from build123d import *

# Parameters (mm, degrees)
BOSS_EXTRUDE1_DEPTH     = 5
SKETCH3_R               = 2.39
BOSS_EXTRUDE2_DEPTH     = 23.4
MIRROR3_COPY_1_SKETCH_R = 2.39
MIRROR3_COPY_1_DEPTH    = 23.4


with BuildPart() as part:
    # Sketch2 → Boss-Extrude1 (new, symmetric)
    with BuildSketch(Plane(origin=(0, 0, 0), x_dir=(1, 0, 0), z_dir=(0, 1, 0))):
        Polygon((-50.18902685, 27.340766285), (-50.18902685, -26.442734497), (-27.080777241, -49.550984106), (26.70272354, -49.550984106), (49.81097315, -26.442734497), (49.81097315, 27.340766285), (26.70272354, 50.449015894), (-27.080777241, 50.449015894), align=None)
    extrude(amount=BOSS_EXTRUDE1_DEPTH, both=True)

    # Sketch3 → Boss-Extrude2 (add)
    with BuildSketch(Plane(origin=(38.126853823, 0, 38.126853823), x_dir=(0.7071067811865475, 0, -0.7071067811865477), z_dir=(0.7071067811865477, 0, 0.7071067811865475))):
        Circle(SKETCH3_R)
    boss_extrude2 = extrude(amount=BOSS_EXTRUDE2_DEPTH)

    # Mirror2: Boss-Extrude2 across plane
    add(boss_extrude2.mirror(Plane(origin=(0, 0, 0), x_dir=(0, 0, 1), z_dir=(1, 0, 0))))

    # Mirror3: Boss-Extrude2 across plane
    add(boss_extrude2.mirror(Plane.XY))

    # Mirror3 copy 1 sketch → Mirror3 copy 1 (add)
    with BuildSketch(Plane(origin=(-38.126853823, 0, -38.126853823), x_dir=(-0.7071067811865475, 0, 0.7071067811865477), z_dir=(-0.7071067811865477, 0, -0.7071067811865475))):
        Circle(MIRROR3_COPY_1_SKETCH_R)
    extrude(amount=MIRROR3_COPY_1_DEPTH)


solid = part.part
Geometry check sheet. Reference: the model listing, model coordinates, mm. A direction names the side the tool comes from. Round coordinates to 2 decimals unless told otherwise and drop trailing zeros. Order: outer loops, then holes, each group sorted by start corner. A loop starts at its lowest first (then second) coordinate and runs counter-clockwise, first axis right, second up. Notation, with made-up numbers: M 69.5,-25 L 126.5,-25 A28 ccw 126.5,2 Z; hole C 14.25,65 d6. An arc over 180 degrees is marked long. Answer in a Markdown table with one row per item. Add a question column.
Item 1: Set-up check for faces 5 (the face through (49.811, 0, 0)), 6 (the face through (-50.189, 0, -1)), 7 (the face through (0, 0, -50.449)), 8 (the face through (-1, 0, 49.551)): record each of +Z, -Z, +X, -X, +Y, -Y from which the full face is reachable in a straight line by a thin tool's end or side.
Item 2: Sectioned sample at C-C, the plane x = -43. State how many separate pieces and enclosed holes the cut face has, plus the area to 3 significant figures.
Item 3: Sectioned sample at B-B, the plane x = 20. Enter the section's corners in (y, z).
Item 4: Draft check along Z on faces 1 (the face through (38.42, 3.4, -38.73)), 2 (the face through (54.649, 0.033, -54.697)), 3 (the face through (-38.47, 3.4, -39.06)), 4 (the face through (-1, 5, -1)). Enter one of: released by +Z, released by -Z, zero draft, split by the parting line, or undercut.
Item 5: Depth check by flat-ended pin: pin 1 Ø1 at (y, z) = (-2.5, 2.5) entering from -X; pin 2 Ø1 at (x, y) = (-44, 0) entering from -Z; pin 3 Ø5 at (x, y) = (-6, 1.5) entering from -Z. Enter the tip coordinate at first touch or a pass-through.
Item 6: Sectioned sample at A-A, the plane z = -25.5. Enter the section's corners in (x, y).
Item 7: Material ranges on L1, parallel to X at y = 2, z = 43.5; L2, parallel to X at y = 2, z = 43; L3, parallel to Z at x = -41.5, y = 1.75, recorded low to high. Write a range as [from, to].
Filled in:
| question | item | result |
|---|---|---|
| 1 | face 5 | +X, +Y, -Y |
| 1 | face 6 | -X, +Y, -Y |
| 1 | face 7 | -Z, +Y, -Y |
| 1 | face 8 | +Z, +Y, -Y |
| 2 | separate pieces | 3 |
| 2 | enclosed holes | 0 |
| 2 | area | 732 mm² |
| 3 | outline | M -5,-50.45 L 5,-50.45 L 5,49.55 L -5,49.55 Z |
| 4 | face 1 | undercut |
| 4 | face 2 | released by -Z |
| 4 | face 3 | undercut |
| 4 | face 4 | zero draft |
| 5 | pin 1 | stops at x = -50.19 |
| 5 | pin 2 | stops at z = -47.88 |
| 5 | pin 3 | stops at z = -50.45 |
| 6 | outline | M -50.19,-5 L 49.81,-5 L 49.81,5 L -50.19,5 Z |
| 7 | L1 | x = [-45.35, -41.65], [-33.13, 32.75], [41.65, 45.35] |
| 7 | L2 | x = [-44.85, -41.15], [-33.63, 33.25], [41.15, 44.85] |
| 7 | L3 | z = [-43.8, -39.2], [-36.03, 35.13], [39.2, 43.8] |
